Part model, mm, in its own coordinate system. A direction names the side the tool comes from. Give positions to 0.01 mm unless a question says otherwise; leave off trailing zeros. Order: outer loops, then holes, each group sorted by start corner. A loop starts at its lowest first (then second) coordinate and runs counter-clockwise, first axis right, second up.
1. Slice it at D-D on x = 25. List the corners of the cut face in (y, z).
2. Slice it at B-B on z = 3.5. List the corners of the cut face in (x, y), and give its area (3 significant figures).
3. Probe line 1 (X direction, y = -10, z = 5.25); line 2 (Y direction, x = -0.5, z = 3.25); line 3 (X direction, y = -12, z = 1.25). List the from-to ranges inside material, lowest first.
4. Slice it at C-C on y = -13. List the corners of the cut face in (x, z).
5. Slice it at A-A on y = 6. List the corners of the cut face in (x, z).
6. Drop a flat-ended pin along its axis: pin 1 Ø1.9 at (x, z) = (-3, 2.5) entering from +Y. Give the stop position or say it passes through.
7. Which spindle directions (+Z, -Z, +X, -X, +Y, -Y) get a long thin tool onto all of the face, cutting with end or side? Do faces 5 (the flat face through (2, -17, 6.35)), 6 (the flat face through (10.859, -2, 3)). Say none if no direction does.
8. Mould opens along X. For faces 1 (the cylindrical face through (39.24, 5.07, 3.13)), 2 (the cylindrical face through (13.31, 10.02, 3.13)), 3 (the cylindrical face through (9.048, -14.349, 3.131)), 4 (the flat face through (2, -17, 0)) say: +X half, -X half, draft (parallel to the pull), parting line (faces both ways), or undercut.
from build123d import *

# Parameters (mm, degrees)
F1_DEPTH = 6.35


with BuildPart() as f1:
    # F0 (on Top) → F1 (new body)
    with BuildSketch(Plane.XY):
        with BuildLine():
            Line((-35.611351, -38.21987), (40.588649, -38.21987))
            Line((40.588649, -38.21987), (40.588649, 1.155555))
            ThreePointArc((40.588649, 1.155555), (39.199232, 5.119784), (35.639008, 7.349221))
            Line((35.639008, 7.349221), (18.609413, 11.199534))
            ThreePointArc((18.609413, 11.199534), (13.244825, 9.966452), (10.859053, 5.005868))
            Line((10.859053, 5.005868), (10.859053, -9.908146))
            ThreePointArc((10.859053, -9.908146), (8.999181, -14.398274), (4.509053, -16.258146))
            Line((4.509053, -16.258146), (-8.190947, -16.258146))
            ThreePointArc((-8.190947, -16.258146), (-12.681075, -14.398274), (-14.540947, -9.908146))
            Line((-14.540947, -9.908146), (-14.540947, 12.951854))
            ThreePointArc((-14.540947, 12.951854), (-19.458817, 27.973251), (-32.308063, 37.177854))
            ThreePointArc((-32.308063, 37.177854), (-34.573491, 36.803467), (-35.611351, 34.755254))
            Line((-35.611351, 34.755254), (-35.611351, -38.21987))
        make_face()
    extrude(amount=F1_DEPTH)


solid = f1.part
Data:
1. outline: (-38.22, 0) - (9.75, 0) - (9.75, 6.35) - (-38.22, 6.35) - close
2. outline: (-35.61, -38.22) - (40.59, -38.22) - (40.59, 1.16) arc R6.35 ccw to (35.64, 7.35) - (18.61, 11.2) arc R6.35 ccw to (10.86, 5.01) - (10.86, -9.91) arc R6.35 cw to (4.51, -16.26) - (-8.19, -16.26) arc R6.35 cw to (-14.54, -9.91) - (-14.54, 12.95) arc R25.4 ccw to (-32.31, 37.18) arc R2.54 ccw to (-35.61, 34.76) - close
2. area: 3,450 mm2
3. line 1: x = -35.61 to -14.54, 10.86 to 40.59
3. line 2: y = -38.22 to -16.26
3. line 3: x = -35.61 to -14.19, 10.5 to 40.59
4. outline: (-35.61, 0) - (-13.74, 0) - (-13.74, 6.35) - (-35.61, 6.35) - close; (10.06, 0) - (40.59, 0) - (40.59, 6.35) - (10.06, 6.35) - close
5. outline: (-35.61, 0) - (-14.54, 0) - (-14.54, 6.35) - (-35.61, 6.35) - close; (10.94, 0) - (38.34, 0) - (38.34, 6.35) - (10.94, 6.35) - close
6. pin 1: stops at y = -16.26
7. face 5: +Z, +X, -X, +Y, -Y
7. face 6: +Z, -Z, +Y
8. face 1: +X half
8. face 2: undercut
8. face 3: undercut
8. face 4: draft
